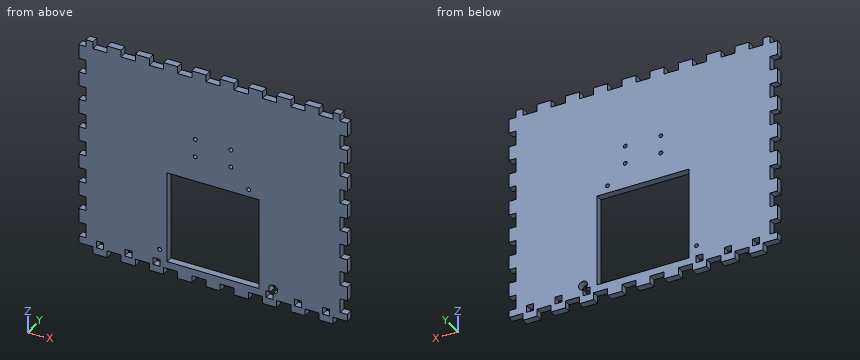
```python
from build123d import *

# Parameters (mm, degrees)
SKETCH1_W            = 241.3
SKETCH1_H            = 254
BOSS_EXTRUDE1_DEPTH  = 6.35
SKETCH2_W            = 6.35
SKETCH2_H            = 12.7
CUT_EXTRUDE1_DEPTH   = 351.402643398
LPATTERN1_COUNT      = 10
LPATTERN1_PITCH      = 25.4
SKETCH3_W            = 12.7
SKETCH3_H            = 6.35
CUT_EXTRUDE2_DEPTH   = 351.402643398
LPATTERN2_COUNT      = 10
LPATTERN2_PITCH      = 25.4
SKETCH4_W            = 241.3
SKETCH4_H            = 57.15
CUT_EXTRUDE3_DEPTH   = 351.402643398
SKETCH5_W            = 12.7
SKETCH5_H            = 6.35
CUT_EXTRUDE4_DEPTH   = 351.402643398
LPATTERN3_COUNT      = 10
LPATTERN3_PITCH      = 25.4
SKETCH6_W            = 82.55
SKETCH6_H            = 82.55
CUT_EXTRUDE5_DEPTH   = 351.402643398
SKETCH7_W            = 6.35
SKETCH7_H            = 6.35
CUT_EXTRUDE6_DEPTH   = 351.402643398
LPATTERN4_COUNT      = 9
LPATTERN4_PITCH      = 25.4
SKETCH8_R            = 1.75
CUT_EXTRUDE7_DEPTH   = 351.402643398
LPATTERN5_COUNT      = 13
LPATTERN5_PITCH      = 16
LPATTERN5_COUNT_DIR2 = 11
LPATTERN5_PITCH_DIR2 = 16
SKETCH9_W            = 48.045746174
SKETCH9_H            = 167.078000208
SKETCH9_W_2          = 46.314367934
SKETCH9_W_3          = 108.643984591
SKETCH9_H_2          = 41.120233212
SKETCH9_W_4          = 31.284165216
SKETCH9_H_3          = 8.622263637
SKETCH9_W_5          = 25.970673607
SKETCH9_H_4          = 10.388269443
SKETCH9_W_6          = 15.149559605
SKETCH9_W_7          = 30.731963769
SKETCH9_W_8          = 73.583575221
SKETCH9_H_5          = 8.656891202
SKETCH9_W_9          = 14.283870484
SKETCH9_W_10         = 8.224046642
SKETCH9_H_6          = 72.285041541
SKETCH9_W_11         = 11.748458615
SKETCH9_H_7          = 59.732549298
SKETCH9_W_12         = 9.178793531
SKETCH9_W_13         = 27.063281488
BOSS_EXTRUDE2_DEPTH  = 6.35
SKETCH10_R           = 3.96875
CUT_EXTRUDE8_DEPTH   = 351.402643398


with BuildPart() as part:
    # Sketch1 → Boss-Extrude1 (new body)
    with BuildSketch(Plane(origin=(0, 0, 0), x_dir=(1, 0, 0), z_dir=(0, 1, 0))):
        with Locations((120.65, 127)):
            Rectangle(SKETCH1_W, SKETCH1_H)
    extrude(amount=BOSS_EXTRUDE1_DEPTH)

    # Sketch2 → Cut-Extrude1 (cut, through all)
    with BuildSketch(Plane(origin=(0, 6.35, 0), x_dir=(1, 0, 0), z_dir=(0, 1, 0))):
        with Locations((3.175, 6.35)):
            Rectangle(SKETCH2_W, SKETCH2_H)
        with Locations((238.125, 6.35)):
            Rectangle(SKETCH2_W, SKETCH2_H)
    cut_extrude1 = extrude(amount=-CUT_EXTRUDE1_DEPTH, mode=Mode.SUBTRACT)

    # LPattern1: Cut-Extrude1 ×10
    with Locations(*[(0, 0, -i * LPATTERN1_PITCH) for i in range(1, LPATTERN1_COUNT)]):
        add(cut_extrude1, mode=Mode.SUBTRACT)

    # Sketch3 → Cut-Extrude2 (cut, through all)
    with BuildSketch(Plane(origin=(0, 6.35, 0), x_dir=(1, 0, 0), z_dir=(0, 1, 0))):
        with Locations((6.35, 3.175)):
            Rectangle(SKETCH3_W, SKETCH3_H)
        with Locations((6.35, 250.825)):
            Rectangle(SKETCH3_W, SKETCH3_H)
    cut_extrude2 = extrude(amount=-CUT_EXTRUDE2_DEPTH, mode=Mode.SUBTRACT)

    # LPattern2: Cut-Extrude2 ×10
    with Locations(*[(i * LPATTERN2_PITCH, 0, 0) for i in range(1, LPATTERN2_COUNT)]):
        add(cut_extrude2, mode=Mode.SUBTRACT)

    # Sketch4 → Cut-Extrude3 (cut, through all)
    with BuildSketch(Plane(origin=(0, 6.35, 0), x_dir=(1, 0, 0), z_dir=(0, 1, 0))):
        with Locations((120.65, 28.575)):
            Rectangle(SKETCH4_W, SKETCH4_H)
    extrude(amount=-CUT_EXTRUDE3_DEPTH, mode=Mode.SUBTRACT)

    # Sketch5 → Cut-Extrude4 (cut, through all)
    with BuildSketch(Plane(origin=(0, 6.35, 0), x_dir=(1, 0, 0), z_dir=(0, 1, 0))):
        with Locations((19.05, 60.325)):
            Rectangle(SKETCH5_W, SKETCH5_H)
    cut_extrude4 = extrude(amount=-CUT_EXTRUDE4_DEPTH, mode=Mode.SUBTRACT)

    # LPattern3: Cut-Extrude4 ×10
    with Locations(*[(i * LPATTERN3_PITCH, 0, 0) for i in range(1, LPATTERN3_COUNT)]):
        add(cut_extrude4, mode=Mode.SUBTRACT)

    # Sketch6 → Cut-Extrude5 (cut, through all)
    with BuildSketch(Plane(origin=(0, 6.35, 0), x_dir=(1, 0, 0), z_dir=(0, 1, 0))):
        with Locations((120.65, 200.025)):
            Rectangle(SKETCH6_W, SKETCH6_H)
    extrude(amount=-CUT_EXTRUDE5_DEPTH, mode=Mode.SUBTRACT)

    # Sketch7 → Cut-Extrude6 (cut, through all)
    with BuildSketch(Plane(origin=(0, 6.35, 0), x_dir=(1, 0, 0), z_dir=(0, 1, 0))):
        with Locations((19.05, 244.475)):
            Rectangle(SKETCH7_W, SKETCH7_H)
    cut_extrude6 = extrude(amount=-CUT_EXTRUDE6_DEPTH, mode=Mode.SUBTRACT)

    # LPattern4: Cut-Extrude6 ×9, 3 skipped
    with Locations(*[(i * LPATTERN4_PITCH, 0, 0) for i in range(1, LPATTERN4_COUNT) if i not in (3, 4, 5)]):
        add(cut_extrude6, mode=Mode.SUBTRACT)

    # Sketch8 → Cut-Extrude7 (cut, through all)
    with BuildSketch(Plane(origin=(0, 6.35, 0), x_dir=(1, 0, 0), z_dir=(0, 1, 0))):
        with Locations(Location((24.65, 72.025, 0), (0, 0, 270))):
            Circle(SKETCH8_R)
    cut_extrude7 = extrude(amount=-CUT_EXTRUDE7_DEPTH, mode=Mode.SUBTRACT)

    # LPattern5: Cut-Extrude7 13 × 11
    with Locations(*[(i * LPATTERN5_PITCH, 0, -j * LPATTERN5_PITCH_DIR2) for i in range(LPATTERN5_COUNT) for j in range(LPATTERN5_COUNT_DIR2) if (i, j) != (0, 0)]):
        add(cut_extrude7, mode=Mode.SUBTRACT)

    # Sketch9 → Boss-Extrude2 (add, through all)
    with BuildSketch(Plane(origin=(0, 6.35, 0), x_dir=(1, 0, 0), z_dir=(0, 1, 0))):
        with Locations((38.409533576, 152.545088079)):
            Rectangle(SKETCH9_W, SKETCH9_H)
        with Locations((203.756155544, 152.545088079)):
            Rectangle(SKETCH9_W_2, SKETCH9_H)
        with Locations((121.948533681, 89.566204581)):
            Rectangle(SKETCH9_W_3, SKETCH9_H_2)
        with Locations((83.268623993, 135.798764893)):
            Rectangle(SKETCH9_W_4, SKETCH9_H_3)
        with Locations((80.611878189, 120.51459063)):
            Rectangle(SKETCH9_W_5, SKETCH9_H_4)
        with Locations((122.814222801, 120.51459063)):
            Rectangle(SKETCH9_W_6, SKETCH9_H_4)
        with Locations((160.904544092, 120.51459063)):
            Rectangle(SKETCH9_W_7, SKETCH9_H_4)
        with Locations((104.418328996, 151.679398959)):
            Rectangle(SKETCH9_W_8, SKETCH9_H_5)
        with Locations((169.128590734, 151.679398959)):
            Rectangle(SKETCH9_W_9, SKETCH9_H_5)
        with Locations((169.128590734, 199.941567413)):
            Rectangle(SKETCH9_W_10, SKETCH9_H_6)
        with Locations((73.500770692, 193.665321291)):
            Rectangle(SKETCH9_W_11, SKETCH9_H_7)
        with Locations((119.828839764, 135.798764893)):
            Rectangle(SKETCH9_W_12, SKETCH9_H_3)
        with Locations((162.738885232, 135.798764893)):
            Rectangle(SKETCH9_W_13, SKETCH9_H_3)
    extrude(amount=-BOSS_EXTRUDE2_DEPTH)

    # Sketch10 → Cut-Extrude8 (cut, through all)
    with BuildSketch(Plane(origin=(0, 6.35, 0), x_dir=(1, 0, 0), z_dir=(0, 1, 0))):
        with Locations((174.625, 238.125)):
            Circle(SKETCH10_R)
    extrude(amount=-CUT_EXTRUDE8_DEPTH, mode=Mode.SUBTRACT)


solid = part.part
```
Read the model definition and answer for the solid it produces. Units are mm, in the model's axes. Round coordinates to 2 decimals unless told otherwise and drop trailing zeros. Write each loop counter-clockwise with the first axis right and the second up, starting at its lowest first coordinate (ties: lowest second). Pieces come first, ordered by that corner, then holes. Notation, with made-up numbers: (0, -33) -> (34, -33) arc R20 ccw to (34, -16) -> close; hole circle Ø5 at (23, -39.5). An arc over 180 degrees is marked (long way). Answer in a Markdown table with one row per item. Add a question column.
1) Find section B-B, the plane y = 4.75. State how many separate pieces and enclosed holes the cut face has, and give its area (3 significant figures).
2) Consider line 1 (Z direction, x = 136.65, y = 3) (3 decimals); line 2 (Z direction, x = 152.65, y = 1.75) (3 decimals); line 3 (Z direction, x = 87, y = 1.25). Determine where each line is inside the solid, lowest interval first.
3) Given P1, Ø3, axis at x = 93, y = 3, coming from the +Z side; P2, Ø3, axis at x = 5.5, y = 2, coming from the -Z side; P3, Ø3, axis at y = 2.5, z = -232.5, coming from the -X side, each flat-ended and moving along its own axis, determine where each tip first touches the part or whether it passes through.
4) Find section A-A, the plane z = -182. Determine the outline of the cut face in (x, y) (3 decimals), and give its area (3 significant figures).
Findings below:
| question | item | result |
|---|---|---|
| 1 | separate pieces | 1 |
| 1 | enclosed holes | 13 |
| 1 | area | 37,600 mm² |
| 2 | line 1 | -247.65 to -241.3, -158.75 to -137.775, -134.275 to -121.775, -118.275 to -57.15 |
| 2 | line 2 | -247.65 to -241.3, -158.75 to -153.775, -150.275 to -57.15 |
| 2 | line 3 | -247.65 to -241.3, -158.75 to -57.15 |
| 3 | P1 | z = -63.5 |
| 3 | P2 | z = -247.65 |
| 3 | P3 | x = 6.35 |
| 4 | outline | (6.35, 0) -> (79.375, 0) -> (79.375, 6.35) -> (6.35, 6.35) -> close; (161.925, 0) -> (234.95, 0) -> (234.95, 6.35) -> (161.925, 6.35) -> close |
| 4 | area | 927 mm² |
